```python
from build123d import *

# Parameters (mm, degrees)
SKETCH1_R           = 55
SKETCH1_R_2         = 37.5
SKETCH1_R_3         = 3.3
BOSS_EXTRUDE1_DEPTH = 3
SKETCH2_R           = 3.175
SKETCH3_R           = 38.7
SKETCH3_R_2         = 37.5
BOSS_EXTRUDE2_DEPTH = 160
SKETCH4_R           = 38.7
BOSS_EXTRUDE3_DEPTH = 3


with BuildPart() as part:
    # Sketch1 → Boss-Extrude1 (new body)
    with BuildSketch(Plane(origin=(0, 0, 0), x_dir=(1, 0, 0), z_dir=(0, 1, 0))):
        Circle(SKETCH1_R)
        Circle(SKETCH1_R_2, mode=Mode.SUBTRACT)
        with Locations((0, 48.6)):
            Circle(SKETCH1_R_3, mode=Mode.SUBTRACT)
        with Locations((46.221346692, 15.018225927)):
            Circle(SKETCH1_R_3, mode=Mode.SUBTRACT)
        with Locations((28.566363261, -39.318225927)):
            Circle(SKETCH1_R_3, mode=Mode.SUBTRACT)
        with Locations((-28.566363261, -39.318225927)):
            Circle(SKETCH1_R_3, mode=Mode.SUBTRACT)
        with Locations((-46.221346692, 15.018225927)):
            Circle(SKETCH1_R_3, mode=Mode.SUBTRACT)
    extrude(amount=BOSS_EXTRUDE1_DEPTH)

    # Sketch2 → Cut-Revolve1 (revolve, cut)
    with BuildSketch(Plane.XY):
        with Locations((40.825, -1.775)):
            Circle(SKETCH2_R)
    revolve(axis=Axis((0, 0, 0), (0, 1, 0)), mode=Mode.SUBTRACT)

    # Sketch3 → Boss-Extrude2 (add)
    with BuildSketch(Plane(origin=(0, 3, 0), x_dir=(1, 0, 0), z_dir=(0, 1, 0))):
        Circle(SKETCH3_R)
        Circle(SKETCH3_R_2, mode=Mode.SUBTRACT)
    extrude(amount=BOSS_EXTRUDE2_DEPTH)

    # Sketch4 → Boss-Extrude3 (add)
    with BuildSketch(Plane(origin=(0, 163, 0), x_dir=(1, 0, 0), z_dir=(0, 1, 0))):
        Circle(SKETCH4_R)
    extrude(amount=BOSS_EXTRUDE3_DEPTH)


solid = part.part
```
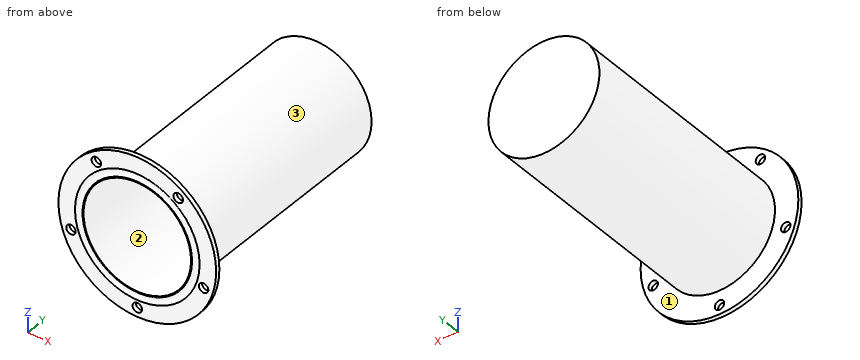
The model under review builds one solid part; all positions refer to its coordinate system, in mm. Face numbers are marked on the shaded views. Give positions to 0.01 mm unless a question says otherwise; leave off trailing zeros. Loops run counter-clockwise (first coordinate to the right, second up) from the corner with the lowest first, then second, coordinate; pieces in that order, holes last. Notation, with made-up numbers: (-16.75, 74.25) - (10.25, 74.25) arc R19 cw to (10.25, 78.25) - close; hole circle Ø6 at (-8.5, -5). An arc over 180 degrees is marked (long way). Answer as a JSON object with one key per item and string values.
Q1. Mouldability with a two-part tool opening along X and no side actions: class the marked faces 1, 2 and 3 as +X half, -X half, draft (parallel to the pull), parting line (faces both ways), or undercut.
Worked out:
{"face 1": "draft", "face 2": "undercut", "face 3": "parting line"}
Q2. Add section D-D on z = -48.6. State the section outline as (x, y) points.
Worked out:
{"outline": "(-25.75, 0) - (-3.3, 0) - (-3.3, 3) - (-25.75, 3) - close; (3.3, 0) - (25.75, 0) - (25.75, 3) - (3.3, 3) - close"}
Q3. Insertion check: pin 1 (6 mm diameter, centred on x = 46.22, z = -15.02, fed in from +Y); pin 2 (7.5 mm diameter, centred on x = 28.57, z = 39.32, fed in from +Y); pin 3 (5 mm diameter, centred on x = 20, y = 102, fed in from -Z); pin 4 (2 mm diameter, centred on x = -19, y = 94.5, fed in from -Z). Each pin has a flat end and moves straight along its axis. Give the tip position at first contact, or say it passes through.
Worked out:
{"pin 1": "passes through", "pin 2": "stops at y = 3", "pin 3": "stops at z = -34.52", "pin 4": "stops at z = -34.26"}
Q4. To check wall thickness, follow line 1 along X through (y, z) = (103, 0); line 2 along X through (y, z) = (11, -30.5). State the ranges of each line that lie inside material, in increasing order.
Worked out:
{"line 1": "x = -38.7 to -37.5, 37.5 to 38.7", "line 2": "x = -23.82 to -21.82, 21.82 to 23.82"}
Q5. Add section C-C on y = 38. State the section outline as (x, z) points.
Worked out:
{"outline": "circle Ø77.4 at (0, 0); hole circle Ø75 at (0, 0)"}
Q6. Add section A-A on x = 0. State the section outline as (y, z) points (3 decimals), plus the area to 3 significant figures.
Worked out:
{"outline": "(0, -55) - (3, -55) - (3, -51.9) - (0, -51.9) - close; (0, -45.3) - (3, -45.3) - (3, -38.7) - (166, -38.7) - (166, 38.7) - (3, 38.7) - (3, 55) - (0, 55) - (0, 43.457) arc R3.175 cw to (0, 38.193) - (0, 37.5) - (163, 37.5) - (163, -37.5) - (0, -37.5) - (0, -38.193) arc R3.175 cw to (0, -43.457) - close", "area": "691 mm^2"}
Q7. Add section B-B on z = 0. State the section outline as (x, y) points (3 decimals), plus the area to 3 significant figures.
Worked out:
{"outline": "(-55, 0) - (-43.457, 0) arc R3.175 cw to (-38.193, 0) - (-37.5, 0) - (-37.5, 163) - (37.5, 163) - (37.5, 0) - (38.193, 0) arc R3.175 cw to (43.457, 0) - (55, 0) - (55, 3) - (38.7, 3) - (38.7, 166) - (-38.7, 166) - (-38.7, 3) - (-55, 3) - close", "area": "711 mm^2"}
